Source: CAD feature listing. Evaluate the final solid. Frame: model axes, mm. Coordinates: 2 decimals unless noted, no trailing zeros. Order: outer loops, then holes, each group sorted by start corner. A loop starts at its lowest first (then second) coordinate and runs counter-clockwise, first axis right, second up.
Item 1: Section B-B on z = 19. Return the cut outline in (x, y).
Item 2: Mould query, pull axis Y, two halves, no side actions, for faces 1 (the flat face through (0, 0, 3)), 2 (the flat face through (0, 0, 0)), 3 (the cylindrical face through (23.846, 7.509, 25.143)). Classes: released by +Y, released by -Y, zero draft, split by the parting line, or undercut.
Item 3: Ray query, line 1 (Y direction, x = 0, z = 27); line 2 (Z direction, x = -9.5, y = 6); line 3 (Y direction, x = 13.5, z = 44). Return the intervals inside material, ascending.
Item 4: Contact query for flat-ended pins moving along their axis: P1, Ø12, axis at x = 13.5, z = 29, coming from the -Y side; P2, Ø1, axis at x = 18.5, y = 16, coming from the +Z side (3 decimals); P3, Ø1.5, axis at x = 1.5, y = -10.5, coming from the +Z side. Output: stop coordinate, or through.
from build123d import *

# Parameters (mm, degrees)
F0_R     = 25
F1_DEPTH = 3
F2_R     = 25
F2_R_2   = 21
F3_DEPTH = 50
F4_R     = 1.99999


# Not quite as in the source:
# - a fillet or chamfer is up to 0.001 mm smaller than in the source, because OpenCascade refuses the exact size


with BuildPart() as f1:
    # F0 (on Top) → F1 (new body)
    with BuildSketch(Plane.XY):
        Circle(F0_R)
    extrude(amount=F1_DEPTH)

    # F2 (on face) → F3 (join)
    with BuildSketch(Plane.XY.offset(3)):
        Circle(F2_R)
        Circle(F2_R_2, mode=Mode.SUBTRACT)
    extrude(amount=F3_DEPTH)

    # F4 (radius 2 in the source; OpenCascade refuses exactly that, so slightly less here)
    f4_edges = [f1.edges().sort_by_distance(p)[0] for p in [
        (-25, 0, 53),
        (-21, 0, 53),
    ]]
    fillet(f4_edges, radius=F4_R)


solid = f1.part
Answer list:
1. outline: circle Ø50 at (0, 0); hole circle Ø42 at (0, 0)
2. face 1: undercut
2. face 2: zero draft
2. face 3: split by the parting line
3. line 1: y = -25 to -21, 21 to 25
3. line 2: z = 0 to 3
3. line 3: y = -21.04 to -16.09, 16.09 to 21.04
4. P1: stops at y = -23.85
4. P2: stops at z = 52.755
4. P3: stops at z = 3
